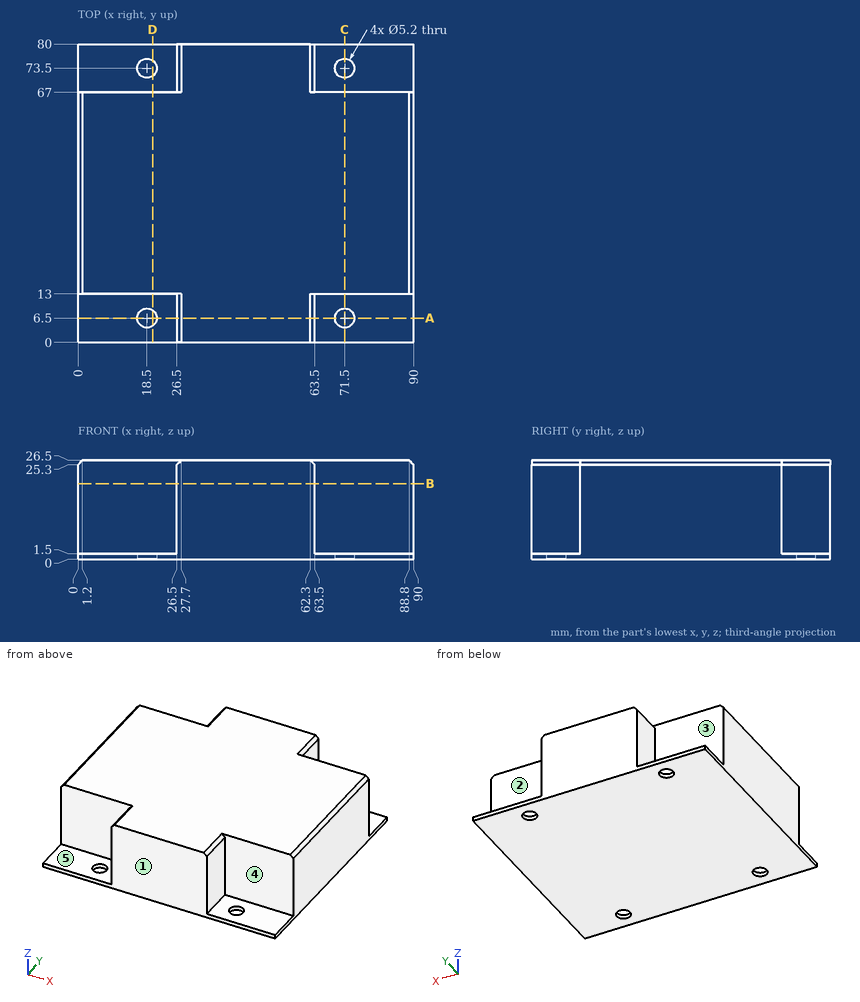
Input: dimensioned drawing with shaded views. Units: mm. Origin: part minimum x, y, z. A direction names the side the tool comes from. Give positions to 0.01 mm unless a question says otherwise; leave off trailing zeros. Loops run counter-clockwise (first coordinate to the right, second up) from the corner with the lowest first, then second, coordinate; pieces in that order, holes last. Notation, with made-up numbers: (1, 85.5) -> (42, 85.5) arc R25 cw to (42, 111.5) -> close; hole circle Ø5 at (48.5, 32.5). An arc over 180 degrees is marked (long way). Return JSON: item names as keys, results as strings.
Item 1: Section A-A, the plane y = 6.5. Output: boundary loops of the cut face in (x, z).
Filled in:
{"outline": "(0, 0) -> (15.9, 0) -> (15.9, 1.5) -> (0, 1.5) -> close; (21.1, 0) -> (68.9, 0) -> (68.9, 1.5) -> (63.5, 1.5) -> (63.5, 25.3) -> (62.3, 26.5) -> (27.7, 26.5) -> (26.5, 25.3) -> (26.5, 1.5) -> (21.1, 1.5) -> close; (74.1, 0) -> (90, 0) -> (90, 1.5) -> (74.1, 1.5) -> close"}
Item 2: Pin query (flat end, axial travel): P1, Ø7.5, axis at x = 82, z = 16.5, coming from the -Y side; P2, Ø6.5, axis at y = 73, z = 8.5, coming from the -X side; P3, Ø4, axis at x = 17, y = 7.5, coming from the +Z side. Return the tip coordinate at first contact, or that it passes through.
Filled in:
{"P1": "y = 13", "P2": "x = 26.5", "P3": "z = 1.5"}
Item 3: Section C-C, the plane x = 71.5. Output: boundary loops of the cut face in (y, z).
Filled in:
{"outline": "(0, 0) -> (3.9, 0) -> (3.9, 1.5) -> (0, 1.5) -> close; (9.1, 0) -> (70.9, 0) -> (70.9, 1.5) -> (67, 1.5) -> (67, 26.5) -> (13, 26.5) -> (13, 1.5) -> (9.1, 1.5) -> close; (76.1, 0) -> (80, 0) -> (80, 1.5) -> (76.1, 1.5) -> close"}
Item 4: Section D-D, the plane x = 20. Output: boundary loops of the cut face in (y, z), plus the area to 3 significant figures.
Filled in:
{"outline": "(0, 0) -> (4.38, 0) -> (4.38, 1.5) -> (0, 1.5) -> close; (8.62, 0) -> (71.38, 0) -> (71.38, 1.5) -> (67, 1.5) -> (67, 26.5) -> (13, 26.5) -> (13, 1.5) -> (8.62, 1.5) -> close; (75.62, 0) -> (80, 0) -> (80, 1.5) -> (75.62, 1.5) -> close", "area": "1,460 mm^2"}
Item 5: Access query for the marked faces 1, 2, 3, 4 and 5. Directions: +Z, -Z, +X, -X, +Y, -Y. A direction counts if a zero-diameter tool reaches every point of the face in a straight line with its end or side. Return the directions, or none.
Filled in:
{"face 1": "+Z, -Z, +X, -X, -Y", "face 2": "+Z, +X, +Y", "face 3": "+Z, -X, +Y", "face 4": "+Z, +X, -Y", "face 5": "+Z, -X, -Y"}
Item 6: Line query: line 1 (Y direction, x = 71.5, z = 0.9); line 2 (Z direction, x = 11.5, y = 73); line 3 (Y direction, x = 16, z = 21). Output: solid intervals per line, ascending.
Filled in:
{"line 1": "0 to 3.9, 9.1 to 70.9, 76.1 to 80", "line 2": "0 to 1.5", "line 3": "13 to 67"}
Item 7: Section B-B, the plane z = 20.25. Output: boundary loops of the cut face in (x, y), plus the area to 3 significant figures.
Filled in:
{"outline": "(0, 13) -> (26.5, 13) -> (26.5, 0) -> (63.5, 0) -> (63.5, 13) -> (90, 13) -> (90, 67) -> (63.5, 67) -> (63.5, 80) -> (26.5, 80) -> (26.5, 67) -> (0, 67) -> close", "area": "5,820 mm^2"}
